Verification items for this drawing (mm, ordinates from the low corner). A direction names the side the tool comes from. Coordinates: 2 decimals unless noted, no trailing zeros. Order: outer loops, then holes, each group sorted by start corner. A loop starts at its lowest first (then second) coordinate and runs counter-clockwise, first axis right, second up. Notation, with made-up numbers: (2, -26) - (11, -26) arc R23 cw to (11, -13) - close; hole circle Ø3 at (45.5, 61). An arc over 180 degrees is marked (long way). Use CSV: the item, a comma, the result in double quotes. Start each with the question number.
1) Depth check by flat-ended pin: P1, Ø1, axis at y = 2.5, z = 4.5, coming from the -X side (1 decimal). Enter the tip coordinate at first touch or a pass-through.
2) Tool access check on the marked faces 4 and 5. Record the directions out of +Z, -Z, +X, -X, +Y, -Y that give a thin tool (end or side, any length) a straight path to the whole face; none if there is none.
3) Sectioned sample at D-D, the plane x = 6.5. Record the cut outline in (y, z).
4) Thickness scan on probe 1 along X at (y, z) = (4.45, 2.5); probe 2 along Z at (x, y) = (4.25, 1.9); probe 3 along Y at (x, z) = (5.5, 4.3). Record the ranges inside material, lowest first. Write a range as [from, to].
5) Sectioned sample at A-A, the plane x = 4.25. Record the cut outline in (y, z), and give its area (3 significant figures).
6) Draft check along X on the marked faces 1, 2 and 3. Enter one of: released by +X, released by -X, zero draft, split by the parting line, or undercut.
7) Sectioned sample at B-B, the plane z = 2.5. Record the cut outline in (x, y).
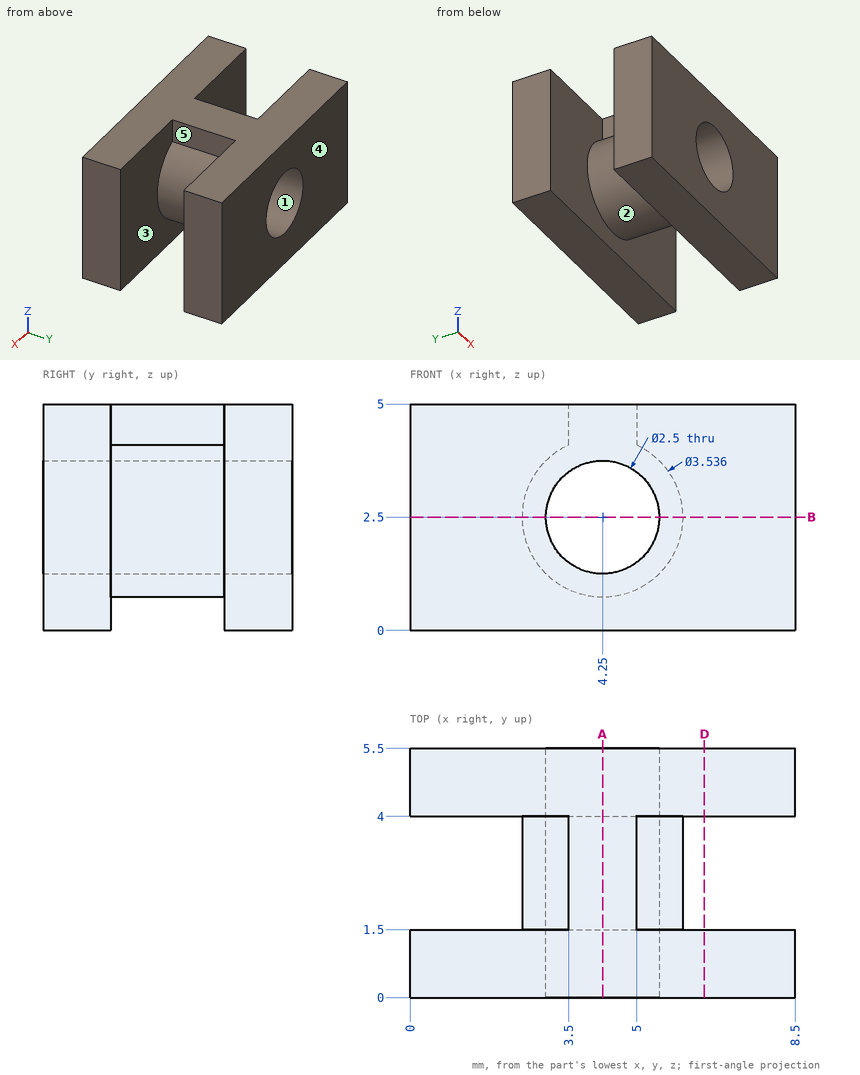
Evaluation:
1,P1,"x = 3.3"
2,face 4,"+Z, -Z, +X, -X, +Y"
2,face 5,"+Z, +X"
3,outline,"(0, 0) - (1.5, 0) - (1.5, 5) - (0, 5) - close; (4, 0) - (5.5, 0) - (5.5, 5) - (4, 5) - close"
4,probe 1,"[0, 3], [5.5, 8.5]"
4,probe 2,"[0.73, 1.25], [3.75, 5]"
4,probe 3,"[0, 1.5], [4, 5.5]"
5,outline,"(0, 0) - (1.5, 0) - (1.5, 0.73) - (4, 0.73) - (4, 0) - (5.5, 0) - (5.5, 1.25) - (0, 1.25) - close; (0, 3.75) - (5.5, 3.75) - (5.5, 5) - (0, 5) - close"
5,area,"11.9 mm²"
6,face 1,"undercut"
6,face 2,"split by the parting line"
6,face 3,"zero draft"
7,outline,"(0, 0) - (3, 0) - (3, 5.5) - (0, 5.5) - (0, 4) - (2.48, 4) - (2.48, 1.5) - (0, 1.5) - close; (5.5, 0) - (8.5, 0) - (8.5, 1.5) - (6.02, 1.5) - (6.02, 4) - (8.5, 4) - (8.5, 5.5) - (5.5, 5.5) - close"
